from build123d import *

# Parameters (mm, degrees)
SKETCH1_W               = 175
SKETCH1_H               = 90
BOSS_EXTRUDE1_DEPTH     = 80
CUT_EXTRUDE4_DEPTH      = 198.610728454
CUT_EXTRUDE4_DEPTH_BACK = 175
SKETCH5_W               = 132.519940576
SKETCH5_H               = 60
CUT_EXTRUDE5_DEPTH      = 175
BOSS_EXTRUDE2_DEPTH     = 20
SKETCH7_R               = 15
SKETCH7_R_2             = 6
CUT_EXTRUDE8_DEPTH      = 20


with BuildPart() as part:
    # Sketch1 → Boss-Extrude1 (new body)
    with BuildSketch(Plane(origin=(0, 0, 0), x_dir=(1, 0, 0), z_dir=(0, 1, 0))):
        Rectangle(SKETCH1_W, SKETCH1_H)
    extrude(amount=BOSS_EXTRUDE1_DEPTH)

    # Sketch4 → Cut-Extrude4 (cut, two sides: drawn at the far end of the back side and taken through both)
    with BuildSketch(Plane.ZY.offset(87.5).offset(-CUT_EXTRUDE4_DEPTH_BACK)):
        Polygon((35, 70), (-35, 70), (-45, 70), (-45, 10), (-35, 10), (35, 10), align=None)
    extrude(amount=CUT_EXTRUDE4_DEPTH + CUT_EXTRUDE4_DEPTH_BACK, mode=Mode.SUBTRACT)

    # Sketch5 → Cut-Extrude5 (cut)
    with BuildSketch(Plane(origin=(0, 80, 0), x_dir=(1, 0, 0), z_dir=(0, 1, 0))):
        with Locations((0, -5)):
            Rectangle(SKETCH5_W, SKETCH5_H)
    extrude(amount=-CUT_EXTRUDE5_DEPTH, mode=Mode.SUBTRACT)

    # Sketch6 → Boss-Extrude2 (add)
    with BuildSketch(Plane(origin=(0, 0, -45), x_dir=(-1, 0, 0), z_dir=(0, 0, -1))):
        with BuildLine():
            Line((-87.5, 0), (-34.003676272, 0))
            ThreePointArc((-34.003676272, 0), (0, -12.5), (34.003676272, 0))
            Line((34.003676272, 0), (87.5, 0))
            Line((87.5, 0), (87.5, 10))
            Line((87.5, 10), (43.084219849, 10))
            ThreePointArc((43.084219849, 10), (52.5, 40), (43.084219849, 70))
            Line((43.084219849, 70), (87.5, 70))
            Line((87.5, 70), (87.5, 80))
            Line((87.5, 80), (34.003676272, 80))
            ThreePointArc((34.003676272, 80), (0, 92.5), (-34.003676272, 80))
            Line((-34.003676272, 80), (-87.5, 80))
            Line((-87.5, 80), (-87.5, 70))
            Line((-87.5, 70), (-43.084219849, 70))
            ThreePointArc((-43.084219849, 70), (-52.5, 40), (-43.084219849, 10))
            Line((-43.084219849, 10), (-87.5, 10))
            Line((-87.5, 10), (-87.5, 0))
        make_face()
    extrude(amount=-BOSS_EXTRUDE2_DEPTH)

    # Sketch7 → Cut-Extrude8 (cut)
    with BuildSketch(Plane(origin=(0, 0, -45), x_dir=(-1, 0, 0), z_dir=(0, 0, -1))):
        with Locations((0, 40)):
            Circle(SKETCH7_R)
        with Locations((40, 40)):
            Circle(SKETCH7_R_2)
        with Locations((24.939592074, 8.726740701)):
            Circle(SKETCH7_R_2)
        with Locations((-8.900837358, 1.002883513)):
            Circle(SKETCH7_R_2)
        with Locations((-36.038754716, 22.644650435)):
            Circle(SKETCH7_R_2)
        with Locations((-36.038754716, 57.355349565)):
            Circle(SKETCH7_R_2)
        with Locations((-8.900837358, 78.997116487)):
            Circle(SKETCH7_R_2)
        with Locations((24.939592074, 71.273259299)):
            Circle(SKETCH7_R_2)
    extrude(amount=-CUT_EXTRUDE8_DEPTH, mode=Mode.SUBTRACT)


solid = part.part
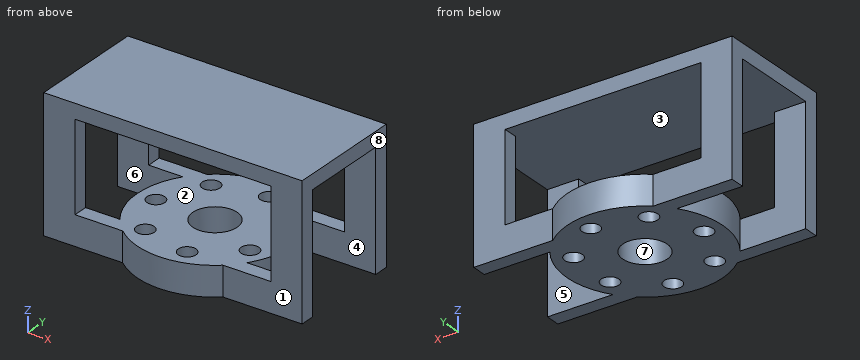
Work out the finished part from the listing and answer in its coordinate system (mm). Face numbers are marked on the shaded views. A direction names the side the tool comes from. Round coordinates to 2 decimals unless told otherwise and drop trailing zeros. Write each loop counter-clockwise with the first axis right and the second up, starting at its lowest first coordinate (ties: lowest second). Pieces come first, ordered by that corner, then holes. Notation, with made-up numbers: M 78,-7 L 119,-7 A15 ccw 119,9 Z; hole C 47.25,3.5 d3. An arc over 180 degrees is marked long. Use a Markdown table: item, result.
1) The part is cut by section C-C on y = 40. Give the vertices of the cut face in (x, z).
Taken from the geometry:
| item | result |
|---|---|
| outline | M -87.5,35 L 87.5,35 L 87.5,45 L -87.5,45 Z; M -52.5,-45 L -46,-45 L -46,-25 L -52.5,-25 Z; M -34,-45 L -15,-45 L -15,-25 L -34,-25 Z; M 15,-45 L 52.5,-45 L 52.5,-25 L 15,-25 Z |
2) Which of the six approach directions +Z, -Z, +X, -X, +Y, -Y give full straight-line access (tool end or side, diameter ignored) to the marked faces 5, 6, 7 and 8?
Taken from the geometry:
| item | result |
|---|---|
| face 5 | -Z, +X |
| face 6 | -Z, -X |
| face 7 | -Z |
| face 8 | +Z, -Z, +X, +Y, -Y |
3) Determine the mould class of the marked faces 1, 2, 3 and 4 for opening direction Y: pulls with the +Y half, pulls with the -Y half, needs draft (parallel to the pull), parting line crosses it, or undercut.
Taken from the geometry:
| item | result |
|---|---|
| face 1 | pulls with the -Y half |
| face 2 | needs draft |
| face 3 | undercut |
| face 4 | undercut |
4) Consider line 1 (Z direction, x = -13, y = 18); line 2 (Y direction, x = 75, z = 0); line 3 (Y direction, x = 0, z = -37.5). Determine where each line is inside the solid, lowest interval first. Write a range as [from, to].
Taken from the geometry:
| item | result |
|---|---|
| line 1 | z = [-45, -25], [35, 45] |
| line 2 | y = [0, 10], [70, 80] |
| line 3 | y = [-12.5, 25], [55, 92.5] |
5) The part is cut by section A-A on z = -1. Give the vertices of the cut face in (x, y), plus the area to 3 significant figures.
Taken from the geometry:
| item | result |
|---|---|
| outline | M -87.5,0 L -66.26,0 L -66.26,10 L -87.5,10 Z; M -87.5,70 L -66.26,70 L -66.26,80 L -87.5,80 Z; M 66.26,0 L 87.5,0 L 87.5,10 L 66.26,10 Z; M 66.26,70 L 87.5,70 L 87.5,80 L 66.26,80 Z |
| area | 850 mm2 |
6) The part is cut by section D-D on z = -33.5. State how many separate pieces and enclosed holes the cut face has, plus the area to 3 significant figures.
Taken from the geometry:
| item | result |
|---|---|
| separate pieces | 1 |
| enclosed holes | 8 |
| area | 9,100 mm2 |
7) The part is cut by section B-B on x = -40. Give the vertices of the cut face in (y, z).
Taken from the geometry:
| item | result |
|---|---|
| outline | M 0,-45 L 34,-45 L 34,-25 L 0,-25 Z; M 0,35 L 80,35 L 80,45 L 0,45 Z; M 46,-45 L 80,-45 L 80,-25 L 46,-25 Z |
8) Flat-ended cylindrical pins translate along their axes: pin 1 (10 mm diameter, centred on x = 57, z = 14, fed in from -Y); pin 2 (13.5 mm diameter, centred on x = 63, z = 13, fed in from +Y); pin 3 (10 mm diameter, centred on y = 12, z = -1.5, fed in from +X); pin 4 (13.5 mm diameter, centred on x = 67, z = -6, fed in from -Y). Find the tip coordinate at first contact, or state that the pin passes through.
Taken from the geometry:
| item | result |
|---|---|
| pin 1 | passes through |
| pin 2 | stops at y = 80 |
| pin 3 | stops at x = 87.5 |
| pin 4 | stops at y = 0 |
